Geometry: final body of the model. Coordinates: model frame, mm. Face numbers are marked on the shaded views. Give positions to 0.01 mm unless a question says otherwise; leave off trailing zeros. Order: outer loops, then holes, each group sorted by start corner. A loop starts at its lowest first (then second) coordinate and runs counter-clockwise, first axis right, second up. Notation, with made-up numbers: (-22, -40) -> (-5, -40) arc R17 cw to (-5, -25) -> close; hole circle Ø3 at (7, 21). An arc over 180 degrees is marked (long way). Answer in a Markdown table with one row per item. Add a question column.
Q1. Cut plane A-A on z = -18. Return the cut outline in (x, y).
Q2. Contact query for flat-ended pins moving along their axis: P1, Ø3, axis at x = -1.5, z = -3.5, coming from the +Y side; P2, Ø2, axis at x = 1.5, z = -10.5, coming from the +Y side; P3, Ø1.5, axis at y = 0, z = -12.5, coming from the -X side; P4, Ø2, axis at x = 2.5, z = -18.5, coming from the -Y side. Output: stop coordinate, or through.
Q3. Pull-direction query (X, two-part tool) for the marked faces 1, 2 and 3; classes: +X half, -X half, draft (parallel to the pull), parting line (faces both ways), or undercut.
Q4. Line query: line 1 along X through (y, z) = (0.5, -1.75); line 2 along Y through (x, z) = (-0.25, -1.5); line 3 along Y through (x, z) = (0, -7.5). Output: solid intervals per line, ascending. Write a range as from..to.
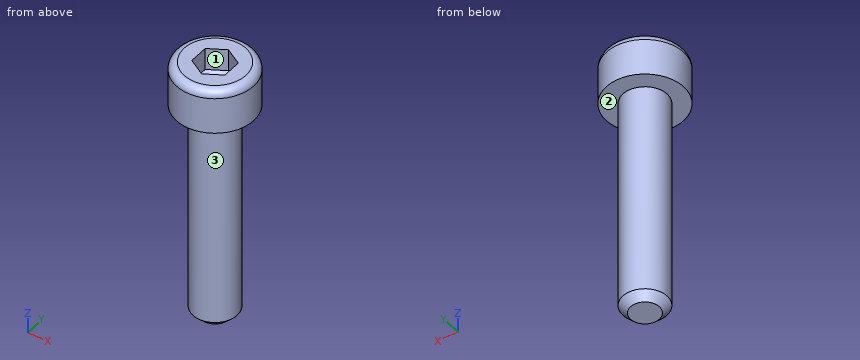
Solid Edge part; units mm, degrees
sketch "Sketch1" plane through (0, 0, 0) normal (0, -1, 0) x (1, 0, 0)
  line L0 (0, 0) -> (2.8, 0)
  arc A0 (2.8, 0) -> (3.5, -0.7) centre (2.8, -0.7) cw
  line L1 (3.5, -0.7) -> (3.5, -4)
  line L2 (3.5, -4) -> (2, -4)
  line L3 (2, -4) -> (2, -23.3)
  line L4 (2, -23.3) -> (1.3, -24)
  line L5 (1.3, -24) -> (0, -24)
revolve "RevolvedProtrusion1" add sketch "Sketch1" angle 360 about axis through (0, 0, -24) along (0, 0, 1)
sketch "Sketch2" plane through (0, 0, 0) normal (0, 0, 1) x (1, 0, 0)
  line L0 (-1.5, -0.866) -> (-1.5, 0.866)
  line L1 (-1.5, 0.866) -> (0, 1.7321)
  line L2 (0, 1.7321) -> (1.5, 0.866)
  line L3 (1.5, 0.866) -> (1.5, -0.866)
  line L4 (1.5, -0.866) -> (0, -1.7321)
  line L5 (0, -1.7321) -> (-1.5, -0.866)
extrude "Cutout1" cut sketch "Sketch2" against normal blind 2
sketch "Sketch3" plane through (0, 0, 0) normal (1, 0, 0) x (0, 1, 0)
  line L0 (0, -3) -> (1.7321, -2)
  line L1 (0, -2) -> (1.7321, -2)
  line L2 (0, -2) -> (0, -3)
revolve "RevolvedCutout1" cut sketch "Sketch3" angle 360 about axis through (0, 0, -60.325) along (0, 0, 1)
cosmetic_thread "Thread1"
Completed:
| question | item | result |
|---|---|---|
| 1 | outline | circle Ø4 at (0, 0) |
| 2 | P1 | stops at y = 3.5 |
| 2 | P2 | stops at y = 1.94 |
| 2 | P3 | stops at x = -2 |
| 2 | P4 | stops at y = -1.32 |
| 3 | face 1 | undercut |
| 3 | face 2 | draft |
| 3 | face 3 | parting line |
| 4 | line 1 | x = -3.46..-1.5, 1.5..3.46 |
| 4 | line 2 | y = -3.49..-1.59, 1.59..3.49 |
| 4 | line 3 | y = -2..2 |
